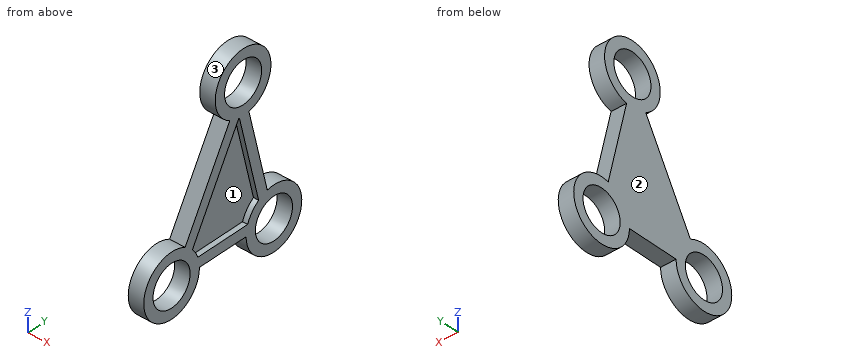
from build123d import *

# Parameters (mm, degrees)
F1_DEPTH = 7.5
F4_DEPTH = 2.5
F5_R     = 15
F6_DEPTH = 7.5
F7_R     = 10
F8_DEPTH = 25


with BuildPart() as f1:
    # F0 (on Right) → F1 (new body)
    with BuildSketch(Plane.YZ):
        Polygon((38.8950196707, 68.8394845703), (0.6499171856, 0), (55.7799171856, 0), align=None)
    extrude(amount=F1_DEPTH)

    # F3 (on offset) → F4 (cut)
    with BuildSketch(Plane.YZ.offset(7.5)):
        Polygon((49.4053139018, 4.9999990523), (37.0754110185, 55.2688359545), (9.1475897815, 4.9999990523), align=None)
    extrude(amount=-F4_DEPTH, mode=Mode.SUBTRACT)

    # F5 (on offset) → F6 (join)
    with BuildSketch(Plane.YZ.offset(7.5)):
        with Locations((39.171077311, 69.5889517665)):
            Circle(F5_R)
        with Locations((55.7799171856, 0)):
            Circle(F5_R)
        with Locations((0.6499171856, 0)):
            Circle(F5_R)
    extrude(amount=-F6_DEPTH)

    # F7 (on offset) → F8 (cut)
    with BuildSketch(Plane.YZ.offset(7.5)):
        with Locations((0.6499171856, 0)):
            Circle(F7_R)
        with Locations((55.7799171856, 0)):
            Circle(F7_R)
        with Locations((39.171077311, 69.5889517665)):
            Circle(F7_R)
    extrude(amount=-F8_DEPTH, mode=Mode.SUBTRACT)


solid = f1.part
Here's how the part is built. I have some questions about the finished solid (model axes, mm). Face numbers are marked on the shaded views. Give positions to 0.01 mm unless a question says otherwise; leave off trailing zeros. Write each loop counter-clockwise with the first axis right and the second up, starting at its lowest first coordinate (ties: lowest second). Pieces come first, ordered by that corner, then holes. Notation, with made-up numbers: (83, 87.25) -> (107, 87.25) arc R19 ccw to (107, 92.25) -> close; hole circle Ø9 at (56, -39.5). An arc over 180 degrees is marked (long way). Use one line per item in the form item = value. Start each with the question number.
1. Will these pins go through, and if not, where does the flat tip stop? pin 1 Ø1.5 at (x, y) = (3.5, 53.5) entering from +Z; pin 2 Ø2 at (x, y) = (5, 27) entering from -Z; pin 3 Ø1.2 at (x, y) = (5.5, 34.5) entering from +Z.
2. If I drill on L1, parallel to Y at x = 3.25, z = -6.5; L2, parallel to Z at x = 5.5, y = 21; L3, parallel to Z at x = 5.5, y = 64, over which ranges is the centre line in solid material (lowest first)?
3. Imagine slicing it at B-B on z = 3.5. List the corners of the cut face in (x, y) for me.
4. Thinking about a two-plate mould opening in Y: for the marked faces 1, 2 and 3, which applies, +Y half, -Y half, draft (parallel to the pull), parting line (faces both ways), or undercut?
5. Imagine slicing it at D-D on x = 1.25. List the corners of the cut face in (y, z) for me.
6. Imagine slicing it at A-A on z = 71.5. List the corners of the cut face in (x, y) for me, plus the area to 3 significant figures.
7. Imagine slicing it at C-C on y = -4. List the corners of the cut face in (x, z) for me.
Entries:
q1.pin_1 = 75.96
q1.pin_2 = 0
q1.pin_3 = 84.03
q2.L1 = -12.87 to -6.95, 8.25 to 14.17, 42.26 to 48.18, 63.38 to 69.3
q2.L2 = 0 to 5, 26.33 to 36.63
q2.L3 = -12.55 to -5.69, 5.69 to 12.55
q3.outline = (0, -13.94) -> (7.5, -13.94) -> (7.5, -8.72) -> (0, -8.72) -> close; (0, 10.02) -> (7.5, 10.02) -> (7.5, 46.41) -> (0, 46.41) -> close; (0, 65.15) -> (7.5, 65.15) -> (7.5, 70.37) -> (0, 70.37) -> close
q4.face_1 = undercut
q4.face_2 = draft
q4.face_3 = parting line
q5.outline = (7.93, 13.11) arc R15 ccw (long way) to (15.65, 0) -> (40.78, 0) arc R15 ccw (long way) to (52.21, 14.57) -> (42.31, 54.92) arc R15 ccw (long way) to (31.99, 56.42) -> close; hole circle Ø20 at (0.65, 0); hole circle Ø20 at (39.17, 69.59); hole circle Ø20 at (55.78, 0)
q6.outline = (0, 24.29) -> (7.5, 24.29) -> (7.5, 29.36) -> (0, 29.36) -> close; (0, 48.99) -> (7.5, 48.99) -> (7.5, 54.05) -> (0, 54.05) -> close
q6.area = 75.9 mm²
q7.outline = (0, -14.26) -> (7.5, -14.26) -> (7.5, -8.85) -> (0, -8.85) -> close; (0, 8.85) -> (7.5, 8.85) -> (7.5, 14.26) -> (0, 14.26) -> close
